Autodesk Inventor part; units mm, degrees
ref_plane "YZ Plane" through (0, 0, 0) normal (1, 0, 0) x (0, 1, 0)
ref_plane "XZ Plane" through (0, 0, 0) normal (0, 1, 0) x (-1, 0, 0)
ref_plane "XY Plane" through (0, 0, 0) normal (0, 0, 1) x (1, 0, 0)
sketch "Sketch1" plane through (0, 0, 0) normal (0, 0, 1) x (1, 0, 0)
  line L0 (0, 0) -> (10, 0)
  line L1 (10, 0) -> (10, 98)
  line L2 (10, 98) -> (0, 98)
  line L3 (0, 98) -> (0, 0)
  line L4 (0, 9.7325) -> (6, 9.7325)
  line L5 (6, 9.7325) -> (6, 6.2675)
  line L6 (6, 6.2675) -> (0, 6.2675)
  line L7 (0, 6.2675) -> (0, 9.7325)
  line L8 (0, 69.7325) -> (6, 69.7325)
  line L9 (6, 69.7325) -> (6, 66.2675)
  line L10 (6, 66.2675) -> (0, 66.2675)
  line L11 (0, 66.2675) -> (0, 69.7325)
  dimension "d0" = 10
  dimension "d1" = 98
  dimension "d10" = 6.2675
  dimension "d11" = 3.465
  dimension "d12" = 6
  dimension "d13" = 3.465
  dimension "d14" = 28.2675
  dimension "d15" = 6
extrude "Extrusion1" add sketch "Sketch1" along normal blind 3
sketch "Sketch2" plane through (0, 0, 3) normal (0, 0, 1) x (1, 0, 0)
  line L0 (10, 0) -> (0, 0)
  line L1 (10, 98) -> (10, 0)
  line L2 (0, 98) -> (10, 98)
  line L3 (6, 3.7) -> (3.5, 3.7)
  line L4 (3.5, 3.7) -> (3.5, 2.3)
  line L5 (3.5, 2.3) -> (6, 2.3)
  line L6 (6, 2.3) -> (6, 3.7)
  line L7 (6, 12.3) -> (3.5, 12.3)
  line L8 (3.5, 12.3) -> (3.5, 13.7)
  line L9 (3.5, 13.7) -> (6, 13.7)
  line L10 (6, 13.7) -> (6, 12.3)
  line L11 (6, 63.7) -> (3.5, 63.7)
  line L12 (3.5, 63.7) -> (3.5, 62.3)
  line L13 (3.5, 62.3) -> (6, 62.3)
  line L14 (6, 62.3) -> (6, 63.7)
  line L15 (6, 72.3) -> (3.5, 72.3)
  line L16 (3.5, 72.3) -> (3.5, 73.7)
  line L17 (3.5, 73.7) -> (6, 73.7)
  line L18 (6, 73.7) -> (6, 72.3)
  dimension "d16" = 1.4
  dimension "d17" = 2.5
  dimension "d18" = 2.3
  dimension "d19" = 1.4
  dimension "d20" = 8.6
  dimension "d21" = 2.5
  dimension "d22" = 4
  dimension "d23" = 1.4
  dimension "d24" = 1.4
  dimension "d25" = 2.5
  dimension "d26" = 24.3
  dimension "d27" = 8.6
extrude "Extrusion2" cut sketch "Sketch2" against normal through all
sketch "草圖7" plane through (0, 0, 3) normal (0, 0, 1) x (1, 0, 0)
  line L0 (0, 98) -> (10, 98)
  point P0 (5, 88)
  point P1 (5, 55)
  dimension "d67" = 10
  dimension "d68" = 43
hole "孔4" at (5, 88, 3) at (5, 55, 3) direction (0, 0, -1) diameter 3 end through all
sketch "草圖8" plane through (0, 0, 3) normal (0, 0, 1) x (1, 0, 0)
  line L0 (0, 0) -> (0, 98)
  line L1 (10, 0) -> (0, 0)
  line L2 (10, 98) -> (10, 0)
  line L3 (0, 98) -> (10, 98)
  circle A0 centre (-7, 49) radius 10
  circle A1 centre (-2, 21.5) radius 7
  circle A2 centre (4, 38.5) radius 3
  line L4 (4, 41.5) -> (0, 41.5)
  line L5 (0, 41.5) -> (0, 35.5)
  line L6 (0, 35.5) -> (4, 35.5)
  line L7 (4, 35.5) -> (4, 41.5)
  point P0 (0, 66.2675)
  point P1 (0, 9.7325)
  dimension "d84" = 6
  dimension "d76" = 49
  dimension "d77" = 7
  dimension "d78" = 20
  dimension "d79" = 12
  dimension "d80" = 21.5
  dimension "d81" = 14
  dimension "d82" = 38.5
  dimension "d83" = 6
extrude "擠出4" cut sketch "草圖8" against normal through all contours L0 L4 A2 L6 | A1 L0 | L0 A1 | L7 A2 | A2 L7 | A0 L0 | L0 A0
fillet "圓角4" radius 2 5 edges at (0, 14.7918, 1.5) (0, 28.2082, 1.5) (0, 35.5, 1.5) (0, 41.5, 1.5) (0, 41.8586, 1.5)
properties part number "plastic_part_53"
Work out the finished part from the listing and answer in its coordinate system (mm). A direction names the side the tool comes from. Coordinates: 2 decimals unless noted, no trailing zeros. Write each loop counter-clockwise with the first axis right and the second up, starting at its lowest first coordinate (ties: lowest second). Pieces come first, ordered by that corner, then holes.
1. The part is cut by section D-D, the plane y = 38.5. Write down the section's boundary in (x, z).
Results list:
outline: (7, 0) - (10, 0) - (10, 3) - (7, 3) - close
2. For a pull along Y with two mould halves and no side action, classify faces 4 (the flat face through (10, 48, 1)), 5 (the cylindrical face through (0.31, 28.49, 1.48)), 6 (the flat face through (5, 98, 1)) as +Y half, -Y half, draft (parallel to the pull), parting line (faces both ways), or undercut.
Results list:
face 4: draft
face 5: undercut
face 6: +Y half
3. For faces 1 (the cylindrical face through (0.292, 14.479, 1.479)), 2 (the flat face through (5, 13.7, 2)), 3 (the flat face through (0, 7, 1)), determine the directions among +Z, -Z, +X, -X, +Y, -Y from which every point of the face is accessible in a straight line to the end or side of a thin tool.
Results list:
face 1: +Z, -Z, -X
face 2: +Z, -Z
face 3: +Z, -Z, -X, +Y, -Y
4. The part is cut by section C-C, the plane y = 55. Write down the section's boundary in (x, z).
Results list:
outline: (1, 0) - (3.5, 0) - (3.5, 3) - (1, 3) - close; (6.5, 0) - (10, 0) - (10, 3) - (6.5, 3) - close
5. The part is cut by section A-A, the plane y = 88. Write down the section's boundary in (x, z).
Results list:
outline: (0, 0) - (3.5, 0) - (3.5, 3) - (0, 3) - close; (6.5, 0) - (10, 0) - (10, 3) - (6.5, 3) - close
6. The part is cut by section B-B, the plane z = 2.45. State how many separate pieces and enclosed holes the cut face has, and give its area (3 significant figures).
Results list:
separate pieces: 1
enclosed holes: 6
area: 830 mm2
7. A flat-ended cylindrical pin translates along its axis: pin 1 (1.8 mm diameter, centred on x = 5, y = 55, fed in from -Z). Find the tip coordinate at first contact, or state that the pin passes through.
Results list:
pin 1: passes through
8. Consider line 1 along X through (y, z) = (88, 1.3); line 2 along X through (y, z) = (13, 1.9); line 3 along X through (y, z) = (50.5, 1.15). Determine where each line is inside the solid, lowest interval first.
Results list:
line 1: x = 0 to 3.5, 6.5 to 10
line 2: x = 0 to 3.5, 6 to 10
line 3: x = 2.89 to 10
